Can you work these out from the model? Positions are in its coordinate system, mm. A direction names the side the tool comes from. Coordinates: 2 decimals unless noted, no trailing zeros. Order: outer loops, then holes, each group sorted by start corner. A loop starts at its lowest first (then second) coordinate and runs counter-clockwise, first axis right, second up. Notation, with made-up numbers: (64, 9.5) - (68, 9.5) arc R29 cw to (68, 47.5) - close; hole circle Ø11 at (8.25, -1.75). An arc over 180 degrees is marked (long way). Use a Markdown table: item, result. Add a question column.
(1) For pin 1 Ø2.5 at (x, z) = (80, 0) entering from -Y; pin 2 Ø3 at (x, y) = (65, -10) entering from +Z; pin 3 Ø2 at (y, z) = (-9, -27.5) entering from -X; pin 4 Ø8 at (x, y) = (65.5, 8) entering from +Z, each with a flat end and sliding along its axis, tell me the tip position at first contact or that it passes through.
(2) I want a section at B-B (x = 80). List the corners of the cut face in (y, z) for me.
(3) On a 3-axis mill with a long thin cutter (end or side, diameter ignored), from which of +Z, -Z, +X, -X, +Y, -Y can I reach the whole of each face in a straight line? I mean faces 1 (the flat face through (75, 12.5, -24)), 2 (the flat face through (70.16, 0.11, -36.19)). Say none if no direction works.
(4) I want a section at A-A (z = -3.5). List the corners of the cut face in (x, y) for me, and give its area (3 significant figures).
(5) If I drill on L1, parallel to Y at x = 68.5, z = -40; L2, parallel to X at y = 0.5, z = -25.5; L3, parallel to Z at x = 68.25, y = 4.5, over which ranges is the centre line in solid material (lowest first)? Write a range as [from, to].
(6) We'd pull the mould along Z, two halves only. Please class faces 3 (the cylindrical face through (80, 0, -10)), 4 (the flat face through (75, -12.5, -24)), 5 (the cylindrical face through (81.586, 10.219, -0.208)), 6 (the cylindrical face through (80.86, 0.18, -26.2)): pulls with the +Z half, pulls with the -Z half, needs draft (parallel to the pull), parting line crosses it, or undercut.
(7) I want a section at D-D (z = -40). List the corners of the cut face in (x, y) for me.
(8) I want a section at C-C (y = -6). List the corners of the cut face in (x, z) for me.
```python
from build123d import *

# Parameters (mm, degrees)
EXTRUDE_1_DEPTH          = 12.5
SKETCH_2_R               = 10
CUT_EXTRUDE_1_DEPTH      = 8
CUT_EXTRUDE_2_DEPTH      = 103.984553477
CUT_EXTRUDE_2_DEPTH_BACK = 103.984553477
SKETCH_3_R               = 1.6


with BuildPart() as part:
    # 草图1 → 凸台-拉伸1 (new, symmetric)
    with BuildSketch(Plane(origin=(0, 0, 0), x_dir=(1, 0, 0), z_dir=(0, 1, 0))):
        with BuildLine():
            ThreePointArc((60.351562504, 44.527394976), (71.243831971, 23.437499997), (75, 0))
            ThreePointArc((75, 0), (80, -5), (85, 0))
            ThreePointArc((85, 0), (80.743009566, 26.5625), (68.3984375, 50.464380979))
            ThreePointArc((68.3984375, 50.464380979), (61.406506999, 51.519325478), (60.351562504, 44.527394976))
        make_face()
    extrude(amount=EXTRUDE_1_DEPTH, both=True)

    # 草图2 → 切除-拉伸1 (cut, symmetric)
    with BuildSketch(Plane(origin=(0, 0, 0), x_dir=(1, 0, 0), z_dir=(0, 1, 0))):
        with Locations((80, 0)):
            Circle(SKETCH_2_R)
        with BuildLine():
            Line((73.420566464, 38.244601007), (66.808461169, 34.082686459))
            ThreePointArc((66.808461169, 34.082686459), (63.794128955, 39.437407507), (60.351562504, 44.527394976))
            ThreePointArc((60.351562504, 44.527394976), (61.406506999, 51.519325478), (68.3984375, 50.464380979))
            ThreePointArc((68.3984375, 50.464380979), (70.215090022, 47.904500135), (71.935985524, 45.279288717))
            Line((71.935985524, 45.279288717), (73.420566464, 38.244601007))
        make_face()
    extrude(amount=CUT_EXTRUDE_1_DEPTH, both=True, mode=Mode.SUBTRACT)

    # 草图3 → 切除-拉伸2 (cut, two sides: drawn at the far end of the back side and taken through both)
    with BuildSketch(Plane(origin=(0, 12.5, 0), x_dir=(1, 0, 0), z_dir=(0, 1, 0)).offset(-CUT_EXTRUDE_2_DEPTH_BACK)):
        with Locations(Location((64.375, 47.49588798, 0), (0, 0, 270))):
            Circle(SKETCH_3_R)
        with Locations(Location((80, 0, 0), (0, 0, 270))):
            Circle(SKETCH_3_R)
    extrude(amount=CUT_EXTRUDE_2_DEPTH + CUT_EXTRUDE_2_DEPTH_BACK, mode=Mode.SUBTRACT)


solid = part.part
```
Answers follow:
| question | item | result |
|---|---|---|
| 1 | pin 1 | passes through |
| 1 | pin 2 | stops at z = -34.68 |
| 1 | pin 3 | stops at x = 69.37 |
| 1 | pin 4 | stops at z = -28.19 |
| 2 | outline | (-12.5, -28.72) - (12.5, -28.72) - (12.5, -1.6) - (8, -1.6) - (8, -10) - (-8, -10) - (-8, -1.6) - (-12.5, -1.6) - close; (-12.5, 1.6) - (-8, 1.6) - (-8, 5) - (-12.5, 5) - close; (8, 1.6) - (12.5, 1.6) - (12.5, 5) - (8, 5) - close |
| 3 | face 1 | +Z, -Z, +X, -X, +Y |
| 3 | face 2 | -X |
| 4 | outline | (74.92, -12.5) - (84.93, -12.5) - (84.93, -8) - (74.92, -8) - close; (74.92, 8) - (84.93, 8) - (84.93, 12.5) - (74.92, 12.5) - close |
| 4 | area | 90.1 mm² |
| 5 | L1 | y = [-12.5, -8], [8, 12.5] |
| 5 | L2 | x = [70.53, 81.08] |
| 5 | L3 | z = [-34.99, -31.1] |
| 6 | face 3 | pulls with the +Z half |
| 6 | face 4 | needs draft |
| 6 | face 5 | undercut |
| 6 | face 6 | pulls with the -Z half |
| 7 | outline | (63.44, -12.5) - (75, -12.5) - (75, 12.5) - (63.44, 12.5) - (63.44, 8) - (73.05, 8) - (73.05, -8) - (63.44, -8) - close |
| 8 | outline | (66.81, -34.08) - (73.42, -38.24) - (71.94, -45.28) arc R85 ccw to (84.53, -8.91) arc R10 cw to (74.53, -8.37) arc R75 cw to start |
